Verification items for the finished model (mm, model axes). Face numbers are marked on the shaded views. A direction names the side the tool comes from. Coordinates: 2 decimals unless noted, no trailing zeros. Write each loop counter-clockwise with the first axis right and the second up, starting at its lowest first coordinate (ties: lowest second). Pieces come first, ordered by that corner, then holes. Notation, with made-up numbers: (25.25, -35) -> (77.25, -35) arc R21 ccw to (77.25, -6) -> close; hole circle Ø7 at (64.25, -11.5). An arc over 180 degrees is marked (long way). Answer in a Markdown table with one row per item.
```python
from build123d import *

# Parameters (mm, degrees)
SKETCH1_W           = 276.225
SKETCH1_H           = 152.4
SKETCH1_W_2         = 273.177
SKETCH1_H_2         = 149.352
BULK_EXTRUDE_DEPTH  = 15.24
FILLET1_R           = 12.7
SHELL_T             = -1.524
SKETCH2_R           = 1.651
BOSS_EXTRUDE3_DEPTH = 50.8


with BuildPart() as part:
    # Sketch1 → Bulk-Extrude (new body)
    with BuildSketch(Plane(origin=(0, 0, 0), x_dir=(1, 0, 0), z_dir=(0, 1, 0))):
        with Locations((136.5885, 74.676)):
            Rectangle(SKETCH1_W, SKETCH1_H)
        with Locations((136.5885, 74.676)):
            Rectangle(SKETCH1_W_2, SKETCH1_H_2, mode=Mode.SUBTRACT)
        with Locations((136.5885, 74.676)):
            Rectangle(SKETCH1_W_2, SKETCH1_H_2)
    extrude(amount=BULK_EXTRUDE_DEPTH)

    # Fillet1
    fillet1_edges = [part.edges().sort_by_distance(p)[0] for p in [
        (136.5885, 15.24, 1.524),
    ]]
    fillet(fillet1_edges, radius=FILLET1_R)

    # Shell
    shell_openings = [part.faces().sort_by_distance(p)[0] for p in [
        (136.5885, 0, -74.676),
    ]]
    offset(amount=SHELL_T, openings=shell_openings, kind=Kind.INTERSECTION)

    # Sketch2 → Boss-Extrude3 (add, symmetric)
    with BuildSketch(Plane(origin=(136.5885, 0, 0), x_dir=(0, 0, -1), z_dir=(1, 0, 0))):
        with BuildLine():
            Line((150.876, 3.175), (150.876, 0))
            ThreePointArc((150.876, 0), (156.29606403, -2.24506403), (154.051, 3.175))
            Line((154.051, 3.175), (150.876, 3.175))
        make_face()
        with Locations((154.051, 0)):
            Circle(SKETCH2_R, mode=Mode.SUBTRACT)
    extrude(amount=BOSS_EXTRUDE3_DEPTH, both=True)


solid = part.part
```
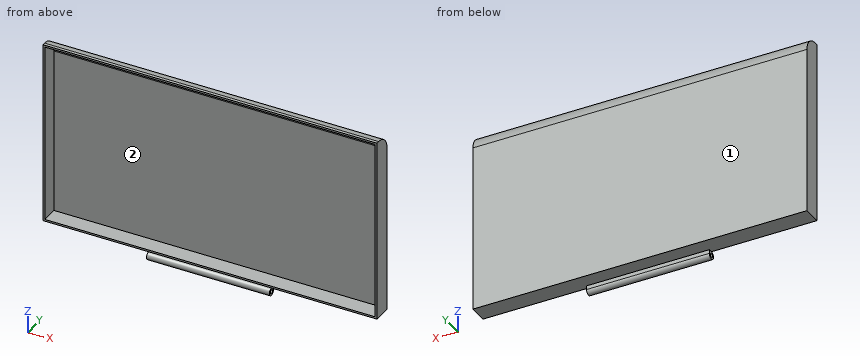
1. Sectioned sample at D-D, the plane x = 57.5. Record the cut outline in (y, z).
Findings below:
| item | result |
|---|---|
| outline | (0, -150.88) -> (15.24, -150.88) -> (15.24, -11.18) arc R12.7 ccw to (2.54, 1.52) -> (0, 1.52) -> (0, 0) -> (2.54, 0) arc R11.18 cw to (13.72, -11.18) -> (13.72, -149.35) -> (0, -149.35) -> close |
2. Sectioned sample at B-B, the plane z = -95.5. Record the cut outline in (x, y), and give its area (3 significant figures).
Findings below:
| item | result |
|---|---|
| outline | (-1.52, 0) -> (0, 0) -> (0, 13.72) -> (273.18, 13.72) -> (273.18, 0) -> (274.7, 0) -> (274.7, 15.24) -> (-1.52, 15.24) -> close |
| area | 463 mm² |
3. Access from +Z, -Z, +X, -X, +Y, -Y to the whole of each face (thin tool, end or side, straight path). Record for the marked faces 1 and 2.
Findings below:
| item | result |
|---|---|
| face 1 | +Z, -Z, +X, -X, +Y |
| face 2 | -Y |
4. Sectioned sample at A-A, the plane x = 169.5. Record the cut outline in (y, z) (3 decimals), and give its area (3 significant figures).
Findings below:
| item | result |
|---|---|
| outline | (0, -150.876) arc R3.175 ccw (long way) to (3.175, -154.051) -> (3.175, -150.876) -> (15.24, -150.876) -> (15.24, -11.176) arc R12.7 ccw to (2.54, 1.524) -> (0, 1.524) -> (0, 0) -> (2.54, 0) arc R11.176 cw to (13.716, -11.176) -> (13.716, -149.352) -> (0, -149.352) -> close; hole circle Ø3.302 at (0, -154.051) |
| area | 292 mm² |
5. Material ranges on probe 1 along Z at (x, y) = (82, 1.75); probe 2 along X at (y, z) = (2.25, -64.5); probe 3 along Z at (x, y) = (129.5, 1.75), recorded low to high. Write a range as from..to.
Findings below:
| item | result |
|---|---|
| probe 1 | z = -150.88..-149.35, 0..1.52 |
| probe 2 | x = -1.52..0, 273.18..274.7 |
| probe 3 | z = -156.7..-149.35, 0..1.52 |
6. Go/stop test with flat-tipped pins: pin 1 (7 mm diameter, centred on y = -0.5, z = -153, fed in from -X); pin 2 (4.5 mm diameter, centred on x = 163.5, y = 8, fed in from -Z); pin 3 (3 mm diameter, centred on y = -1, z = -153.5, fed in from +X); pin 4 (2 mm diameter, centred on x = 26.5, y = 12.5, fed in from +Z). Record where each tip stops, or that it passes through.
Findings below:
| item | result |
|---|---|
| pin 1 | stops at x = -1.52 |
| pin 2 | stops at z = -150.88 |
| pin 3 | stops at x = 187.39 |
| pin 4 | stops at z = -2.18 |
7. Sectioned sample at C-C, the plane y = 6. Record the cut outline in (x, z).
Findings below:
| item | result |
|---|---|
| outline | (-1.52, -150.88) -> (274.7, -150.88) -> (274.7, 1.04) -> (-1.52, 1.04) -> close; hole (0, -149.35) -> (273.18, -149.35) -> (273.18, -0.55) -> (0, -0.55) -> close |
